Can you work these out from the model? Positions are in its coordinate system, mm. Face numbers are marked on the shaded views. A direction names the side the tool comes from. Round coordinates to 2 decimals unless told otherwise and drop trailing zeros. Loops run counter-clockwise (first coordinate to the right, second up) from the corner with the lowest first, then second, coordinate; pieces in that order, holes last. Notation, with made-up numbers: (74, 69.25) -> (111, 69.25) arc R38 cw to (111, 108.25) -> close; hole circle Ø9 at (20.25, 60). An arc over 180 degrees is marked (long way). Write item = value, one per line.
from build123d import *

# Parameters (mm, degrees)
F0_R     = 4
F1_DEPTH = 11
F3_DEPTH = 5
F6_D     = 4
F6_DEPTH = 8
F6_TIP   = 1.2017212381


with BuildPart() as f1:
    # F0 (on Top) → F1 (new body)
    with BuildSketch(Plane.XY):
        Circle(F0_R)
    extrude(amount=F1_DEPTH)

    # F2 (on Top) → F3 (join)
    with BuildSketch(Plane.XY):
        Polygon((0.8915454574, -6.4456966717), (6.0279097915, -2.4507473211), (5.1363643341, 3.9949493506), (-0.8915454574, 6.4456966717), (-6.0279097915, 2.4507473211), (-5.1363643341, -3.9949493506), align=None)
    extrude(amount=F3_DEPTH)

    # F6
    with Locations(Plane.XY.offset(11)):
        with Locations((0, 0)):
            Hole(F6_D / 2, depth=F6_DEPTH)
            with Locations((0, 0, -(F6_DEPTH + F6_TIP / 2))):  # 118° drill point
                Cone(0, F6_D / 2, F6_TIP, mode=Mode.SUBTRACT)


solid = f1.part
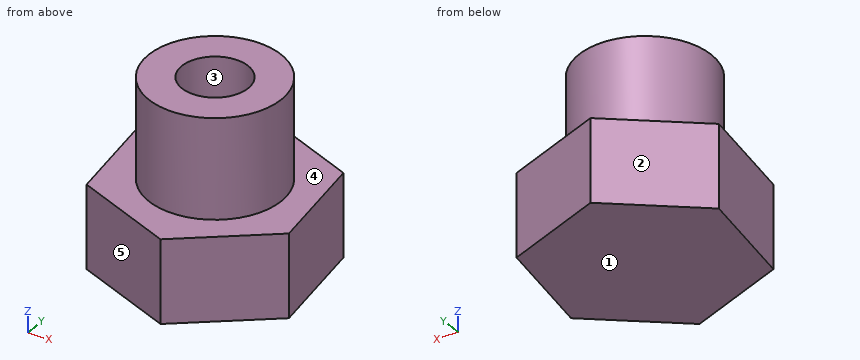
1. Suppose I cut it at D-D, the plane z = 6. List the corners of the cut face in (x, y) for me.
Entries:
outline = circle Ø8 at (0, 0); hole circle Ø4 at (0, 0)
2. Suppose I cut it at A-A, the plane z = 3.5. List the corners of the cut face in (x, y) for me, and give its area (3 significant figures).
Entries:
outline = (-6.03, 2.45) -> (-5.14, -3.99) -> (0.89, -6.45) -> (6.03, -2.45) -> (5.14, 3.99) -> (-0.89, 6.45) -> close; hole circle Ø4 at (0, 0)
area = 97.4 mm²
3. I'm going to push flat-ended pins straight in: pin 1 (3 mm diameter, centred on y = -4.5, z = 7, fed in from -X); pin 2 (6 mm diameter, centred on x = -3, z = 6, fed in from +Y); pin 3 (6 mm diameter, centred on x = 3, z = 9, fed in from +Y); pin 4 (1.5 mm diameter, centred on y = -4, z = 3.5, fed in from -X). Where does each tip first touch, or does it pass through?
Entries:
pin_1 = -2.65
pin_2 = 6.45
pin_3 = 4
pin_4 = -5.24
4. Suppose I cut it at C-C, the plane y = 3.5. List the corners of the cut face in (x, z) for me, and give its area (3 significant figures).
Entries:
outline = (-4.68, 0) -> (5.2, 0) -> (5.2, 5) -> (1.94, 5) -> (1.94, 11) -> (-1.94, 11) -> (-1.94, 5) -> (-4.68, 5) -> close
area = 72.7 mm²
5. I need wall thicknesses on line 1 (Y direction, x = 0, z = 6.25); line 2 (Z direction, x = -2, y = 4.5). Which ranges of each line are inside material? Lowest first, please. Write a range as [from, to].
Entries:
line_1 = [-4, -2], [2, 4]
line_2 = [0, 5]
6. We'd pull the mould along X, two halves only. Please class the marked faces 1, 2 and 3: released by +X, released by -X, zero draft, split by the parting line, or undercut.
Entries:
face_1 = zero draft
face_2 = released by -X
face_3 = undercut
7. For the marked faces 4 and 5, which set-ups out of +Z, -Z, +X, -X, +Y, -Y let a thin tool reach every point of the face, with its end or its side?
Entries:
face_4 = +Z
face_5 = +Z, -Z, -X, -Y
8. Suppose I cut it at B-B, the plane x = 3. List the corners of the cut face in (y, z) for me.
Entries:
outline = (-4.81, 0) -> (4.86, 0) -> (4.86, 5) -> (2.65, 5) -> (2.65, 11) -> (-2.65, 11) -> (-2.65, 5) -> (-4.81, 5) -> close
